Verification items for the finished model (mm, model axes). Coordinates: 2 decimals unless noted, no trailing zeros. Loops run counter-clockwise (first coordinate to the right, second up) from the corner with the lowest first, then second, coordinate; pieces in that order, holes last.
Q1. Sectioned sample at B-B (y = -73.25). Enter the section's corners in (x, z), then the cut area to 3 significant figures.
Q2. Sectioned sample at A-A (z = 0). Enter the section's corners in (x, y) (3 decimals).
Q3. Sectioned sample at D-D (y = 80). Enter the section's corners in (x, z) (3 decimals).
Q4. Sectioned sample at C-C (x = 3.25). Enter the section's corners in (y, z) (3 decimals), then the cut area to 3 significant figures.
Q5. Material ranges on probe 1 along Y at (x, z) = (1, -41); probe 2 along Y at (x, z) = (2.25, -12.5); probe 3 along Y at (x, z) = (6, 10), recorded low to high.
```python
from build123d import *

# Parameters (mm, degrees)
SKETCH1_W           = 101.6
SKETCH1_H           = 210
SKETCH1_R           = 2.1
SKETCH1_R_2         = 14.275
BOSS_EXTRUDE1_DEPTH = 6.35


with BuildPart() as part:
    # Sketch1 → Boss-Extrude1 (new body)
    with BuildSketch(Plane(origin=(0, 0, 0), x_dir=(0, 0, -1), z_dir=(1, 0, 0))):
        Rectangle(SKETCH1_W, SKETCH1_H)
        with Locations((-40.513, -98.65)):
            Circle(SKETCH1_R, mode=Mode.SUBTRACT)
        with Locations((40.513, -98.65)):
            Circle(SKETCH1_R, mode=Mode.SUBTRACT)
        with Locations((0, 80)):
            Circle(SKETCH1_R_2, mode=Mode.SUBTRACT)
        with Locations((-40.513, -73.25)):
            Circle(SKETCH1_R, mode=Mode.SUBTRACT)
        with Locations((40.513, -73.25)):
            Circle(SKETCH1_R, mode=Mode.SUBTRACT)
    extrude(amount=BOSS_EXTRUDE1_DEPTH)


solid = part.part
```
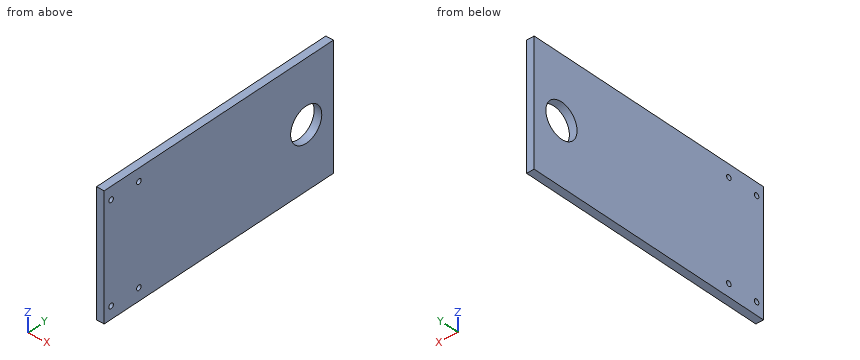
Geometry check:
1. outline: (0, -50.8) - (6.35, -50.8) - (6.35, -42.61) - (0, -42.61) - close; (0, -38.41) - (6.35, -38.41) - (6.35, 38.41) - (0, 38.41) - close; (0, 42.61) - (6.35, 42.61) - (6.35, 50.8) - (0, 50.8) - close
1. area: 592 mm2
2. outline: (0, -105) - (6.35, -105) - (6.35, 65.725) - (0, 65.725) - close; (0, 94.275) - (6.35, 94.275) - (6.35, 105) - (0, 105) - close
3. outline: (0, -50.8) - (6.35, -50.8) - (6.35, -14.275) - (0, -14.275) - close; (0, 14.275) - (6.35, 14.275) - (6.35, 50.8) - (0, 50.8) - close
4. outline: (-105, -50.8) - (105, -50.8) - (105, 50.8) - (-105, 50.8) - close; hole circle Ø4.2 at (-98.65, -40.513); hole circle Ø4.2 at (-98.65, 40.513); hole circle Ø4.2 at (-73.25, -40.513); hole circle Ø4.2 at (-73.25, 40.513); hole circle Ø28.55 at (80, 0)
4. area: 20,600 mm2
5. probe 1: y = -105 to -100.69, -96.61 to -75.29, -71.21 to 105
5. probe 2: y = -105 to 73.11, 86.89 to 105
5. probe 3: y = -105 to 69.81, 90.19 to 105
